Autodesk Inventor part; units mm, degrees
ref_plane "Work Plane1" through (0, 0, 10.287) normal (0, 0, -1) x (-1, 0, 0)
ref_plane "YZ Plane" through (0, 0, 0) normal (1, 0, 0) x (0, 1, 0)
ref_plane "XZ Plane" through (0, 0, 0) normal (0, 1, 0) x (-1, 0, 0)
sketch "Sketch1" plane through (0, 0, 0) normal (0, 0, 1) x (1, 0, 0)
  line L0 (0, 0) -> (38.1, 0)
  line L1 (38.1, 0) -> (38.1, 16.2033)
  line L2 (0, 50.8) -> (0, 0)
  line L3 (0, 50.8) -> (13.5942, 58.6486)
  line L4 (0, 50.8) -> (12.7, 28.803)
  line L5 (12.7, 28.803) -> (26.2942, 36.6516)
  line L6 (26.2942, 36.6516) -> (13.5942, 58.6486)
  line L7 (26.2942, 36.6516) -> (38.1, 16.2033)
  dimension "d0" = 15.6972
  dimension "d1" = 25.4
  dimension "d2" = 38.1
  dimension "d3" = 50.8
  dimension "d4" = 120
extrude "Extrusion1" add sketch "Sketch1" along normal blind 20.574 contours L2 L4 L5 L7 L1 L0
sketch "Sketch2" plane through (0, 0, 20.574) normal (0, 0, 1) x (1, 0, 0)
  line L0 (0, 50.8) -> (0, 0)
  line L1 (0, 0) -> (38.1, 0)
  line L2 (38.1, 0) -> (38.1, 16.2033)
  line L3 (38.1, 16.2033) -> (26.2942, 36.6516)
  line L4 (26.2942, 36.6516) -> (12.7, 28.803)
  line L5 (12.7, 28.803) -> (0, 50.8)
  line L6 (26.2942, 36.6516) -> (13.5942, 58.6486)
  line L7 (13.5942, 58.6486) -> (0, 50.8)
  line L8 (38.1, 16.2033) -> (26.2942, 36.6516)
extrude "Extrusion2" add sketch "Sketch2" along normal blind 2.54
ref_plane "Work Plane1" through (0, 0, 10.287) normal (0, 0, -1) x (-1, 0, 0)
mirror "Mirror1" about plane through (0, 0, 10.287) normal (0, 0, -1) of "Extrusion2"
sketch "Sketch3" plane through (0, 0, 23.114) normal (0, -1, 0) x (1, 0, 0)
  line L0 (38.1, -25.654) -> (38.1, 0)
  line L1 (38.1, -6.477) -> (33.02, -6.477)
  line L2 (33.02, -6.477) -> (33.02, -19.177)
  line L3 (33.02, -19.177) -> (38.1, -19.177)
  line L4 (38.1, -19.177) -> (38.1, -6.477)
  point P0 (0, -23.114)
  point P1 (38.1, -12.827)
  point P2 (38.1, -19.177)
  dimension "d9" = 12.7
  dimension "d10" = 5.08
  dimension "d11" = 6.35
extrude "Extrusion3" cut sketch "Sketch3" against normal blind 33.9725
sketch "Sketch4" plane through (33.02, 0, 16.637) normal (1, 0, 0) x (0, 0, -1)
  circle A0 centre (6.35, 7.422) radius 1.778
  point P0 (16.637, 0)
extrude "Extrusion4" cut sketch "Sketch4" against normal blind 15.24
ref_plane "Work Plane2" through (0, 0, 10.287) normal (0, 0, 1) x (1, 0, 0)
sketch "Sketch5" plane through (0, 0, 10.287) normal (0, 0, 1) x (1, 0, 0)
  line L0 (26.2942, 36.6516) -> (12.7, 28.803)
  line L1 (16.51, 31.0027) -> (11.43, 31.0027)
  line L2 (12.7, 28.803) -> (0, 50.8)
  line L3 (16.51, 31.0027) -> (16.51, 0)
  line L4 (0, 0) -> (38.1, 0)
  line L5 (11.43, 31.0027) -> (11.43, 0)
  line L6 (16.51, 0) -> (11.43, 0)
  dimension "d16" = 5.08
extrude "Extrusion5" cut sketch "Sketch5" along normal mid plane 10.16 contours L3 L4 L5 L2 L0
sketch "Sketch6" plane through (13.5942, 58.6486, 23.114) normal (0.8660254, 0.5, 0) x (0, 0, -1)
  line L0 (23.114, -25.4) -> (2.54, -25.4)
  line L1 (2.54, -25.4) -> (2.54, -37.7698)
  line L2 (2.54, -37.7698) -> (23.114, -37.7698)
  line L3 (23.114, -37.7698) -> (23.114, -25.4)
  point P0 (23.114, -43.9941)
  dimension "d19" = 12.3698
extrude "Extrusion6" cut sketch "Sketch6" against normal blind 5.08
chamfer "Chamfer1" distance 1.016 angle 45 1 edges at (21.893, 34.1106, 10.287)
sketch "Sketch7" plane through (9.1948, 56.1086, 23.114) normal (0.8660254, 0.5, 0) x (0, 0, -1)
  circle A0 centre (12.827, -31.5849) radius 1.778
  line L0 (2.54, -25.4) -> (2.54, -26.416)
  line L1 (2.54, -37.7698) -> (2.54, -26.416)
  line L2 (23.114, -37.7698) -> (2.54, -37.7698)
  line L3 (2.54, -25.4) -> (2.54, -37.7698)
  line L4 (2.54, -25.4) -> (2.54, -37.7698)
  point P0 (23.114, -43.9941)
  point P1 (2.54, -31.5849)
  point P2 (12.827, -37.7698)
  dimension "d25" = 3.556
extrude "Extrusion7" cut sketch "Sketch7" against normal blind 7.62
sketch "Sketch8" plane through (0, 0, 23.114) normal (-1, 0, 0) x (0, 0, 1)
  circle A0 centre (-12.827, 19.05) radius 1.778
  point P0 (-23.114, 0)
extrude "Extrusion8" cut sketch "Sketch8" against normal blind 15.24
sketch "Sketch9" plane through (0, 0, 23.114) normal (0, -1, 0) x (1, 0, 0)
  circle A0 centre (5.08, -12.827) radius 1.778
  circle A1 centre (22.86, -6.35) radius 1.778
  circle A2 centre (22.86, -6.35) radius 1.778
  circle A3 centre (5.08, -12.827) radius 1.778
  point P0 (0, -23.114)
extrude "Extrusion9" cut sketch "Sketch9" against normal blind 15.24
properties part number "PALM 1"
Verification items for the finished model (mm, model axes). A direction names the side the tool comes from. Coordinates: 2 decimals unless noted, no trailing zeros. Write each loop counter-clockwise with the first axis right and the second up, starting at its lowest first coordinate (ties: lowest second). Pieces come first, ordered by that corner, then holes. Notation, with made-up numbers: (-14, 81) -> (31, 81) arc R11 cw to (31, 96) -> close; hole circle Ø11 at (43.25, 55). An arc over 180 degrees is marked (long way). One line per item, written item: value. Start each with the question number.
Q1. Cross-section at B-B on z = 1.75. Enter the section's corners in (x, y), and give its area (3 significant figures).
Q2. Mould release check, pull along X, two halves, no side actions. Record for faces 5 (the flat face through (6.89, 54.78, 21.83)), 6 (the flat face through (38.1, 8, 1)), 7 (the cylindrical face through (21.47, 27.34, 8.59)), 8 (the cylindrical face through (3.77, 7.51, 11.49)): pulls with the +X half, pulls with the -X half, needs draft (parallel to the pull), parting line crosses it, or undercut.
Q3. Go/stop test with flat-tipped pins: P1, Ø1.1, axis at x = 23, z = 16.5, coming from the -Y side; P2, Ø5.5, axis at x = 5.08, z = 10.287, coming from the +Y side; P3, Ø1, axis at y = 38, z = 18.5, coming from the +X side. Record where each tip stops, or that it passes through.
Q4. Cross-section at C-C on x = 31.5. Enter the section's corners in (y, z), and give its area (3 significant figures).
Q5. Cross-section at A-A on y = 12.5. Enter the section's corners in (x, z), and give its area (3 significant figures).
Q6. Access from +Z, -Z, +X, -X, +Y, -Y to the whole of each face (thin tool, end or side, straight path). Record for faces 1 (the cylindrical face through (5.635, 20.813, 10.056)), 2 (the flat face through (33.02, 12, 10)), 3 (the cylindrical face through (22.47, 7.51, 15.03)), 4 (the flat face through (21.717, 33.414, 10.143)).
Q7. Cross-section at D-D on y = 43. Enter the section's corners in (x, z), and give its area (3 significant figures).
Q8. Thickness scan on L1, parallel to Z at x = 11, y = 32; L2, parallel to X at y = 8.5, z = 9; L3, parallel to Y at x = 23, z = 10.25. Record the ranges inside material, lowest first. Write a range as from..to.
Checked values:
1. outline: (0, 0) -> (38.1, 0) -> (38.1, 16.2) -> (32.48, 25.94) -> (28.08, 23.4) -> (22.4, 33.23) -> (21.01, 33.6) -> (12.7, 28.8) -> (0, 50.8) -> close
1. area: 1,200 mm²
2. face 5: pulls with the -X half
2. face 6: pulls with the +X half
2. face 7: undercut
2. face 8: undercut
3. P1: stops at y = 15.24
3. P2: stops at y = 46.76
3. P3: stops at x = 7.68
4. outline: (0, -2.54) -> (27.63, -2.54) -> (27.63, 0) -> (25.37, 0) -> (25.37, 20.57) -> (27.63, 20.57) -> (27.63, 23.11) -> (0, 23.11) -> close; hole circle Ø3.56 at (7.42, 10.29)
4. area: 652 mm²
5. outline: (0, -2.54) -> (38.1, -2.54) -> (38.1, 3.94) -> (33.02, 3.94) -> (33.02, 16.64) -> (38.1, 16.64) -> (38.1, 23.11) -> (0, 23.11) -> close; hole circle Ø3.56 at (5.08, 10.29); hole (11.43, 5.21) -> (16.51, 5.21) -> (16.51, 15.37) -> (11.43, 15.37) -> close; hole circle Ø3.56 at (22.86, 16.76)
5. area: 841 mm²
6. face 1: -X
6. face 2: +X, +Y, -Y
6. face 3: -Y
6. face 4: +X, +Y
7. outline: (0, -2.54) -> (22.63, -2.54) -> (22.63, 0) -> (4.5, 0) -> (4.5, 20.57) -> (22.63, 20.57) -> (22.63, 23.11) -> (0, 23.11) -> close
7. area: 208 mm²
8. L1: z = -2.54..0, 20.57..23.11
8. L2: x = 0..3.85, 6.31..11.43, 16.51..17.78
8. L3: y = 0..5.64, 9.2..25.56, 29.66..32.19
